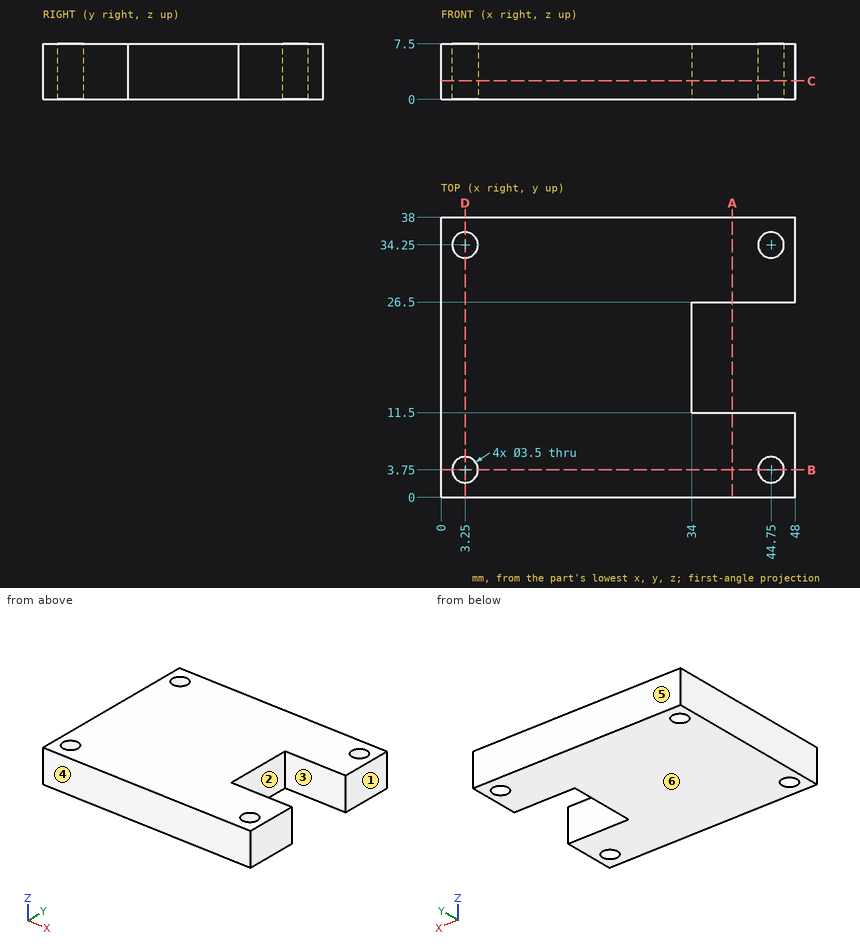
Answer from the drawing. Dimensions are ordinates in mm from the lowest x, y and z of the part. A direction names the side the tool comes from. Round coordinates to 2 decimals unless told otherwise and drop trailing zeros. Order: outer loops, then holes, each group sorted by start corner. A loop starts at its lowest first (then second) coordinate and runs counter-clockwise, first axis right, second up. Notation, with made-up numbers: (85.5, 27.5) - (123.5, 27.5) arc R21 cw to (123.5, 56.5) - close; hole circle Ø1 at (-6, 78). An arc over 180 degrees is marked (long way). Put each result on its own line as item: value. Start each with the question number.
(1) Find section A-A (x = 39.5). Give the vertices of the cut face in (y, z), plus the area to 4 significant figures.
(2) Find section B-B (y = 3.75). Give the vertices of the cut face in (x, z), plus the area to 4 significant figures.
(3) For the marked faces 1 and 2, determine the directions among +Z, -Z, +X, -X, +Y, -Y from which every point of the face is accessible in a straight line to the end or side of a thin tool.
(4) Determine the mould class of the marked faces 3, 4, 5 and 6 for opening direction Y: released by +Y, released by -Y, zero draft, split by the parting line, or undercut.
(5) Straight lines are drawn through the part: probe 1 along Y at (x, z) = (3.25, 2.5); probe 2 along Y at (x, z) = (44.5, 4); probe 3 along X at (y, z) = (2.5, 5.75). For each, find the intervals that lie inside material, in ascending order. Write a range as from..to.
(6) Find section C-C (z = 2.5). Give the vertices of the cut face in (x, y), plus the area to 3 significant figures.
(7) Find section D-D (x = 3.25). Give the vertices of the cut face in (y, z), plus the area to 4 significant figures.
Reply:
1. outline: (0, 0) - (11.5, 0) - (11.5, 7.5) - (0, 7.5) - close; (26.5, 0) - (38, 0) - (38, 7.5) - (26.5, 7.5) - close
1. area: 172.5 mm^2
2. outline: (0, 0) - (1.5, 0) - (1.5, 7.5) - (0, 7.5) - close; (5, 0) - (43, 0) - (43, 7.5) - (5, 7.5) - close; (46.5, 0) - (48, 0) - (48, 7.5) - (46.5, 7.5) - close
2. area: 307.5 mm^2
3. face 1: +Z, -Z, +X, +Y, -Y
3. face 2: +Z, -Z, +X
4. face 3: undercut
4. face 4: released by -Y
4. face 5: released by +Y
4. face 6: zero draft
5. probe 1: 0..2, 5.5..32.5, 36..38
5. probe 2: 0..2.02, 5.48..11.5, 26.5..32.52, 35.98..38
5. probe 3: 0..2.03, 4.47..43.53, 45.97..48
6. outline: (0, 0) - (48, 0) - (48, 11.5) - (34, 11.5) - (34, 26.5) - (48, 26.5) - (48, 38) - (0, 38) - close; hole circle Ø3.5 at (3.25, 3.75); hole circle Ø3.5 at (3.25, 34.25); hole circle Ø3.5 at (44.75, 3.75); hole circle Ø3.5 at (44.75, 34.25)
6. area: 1,580 mm^2
7. outline: (0, 0) - (2, 0) - (2, 7.5) - (0, 7.5) - close; (5.5, 0) - (32.5, 0) - (32.5, 7.5) - (5.5, 7.5) - close; (36, 0) - (38, 0) - (38, 7.5) - (36, 7.5) - close
7. area: 232.5 mm^2
